Can you work these out from the model? Positions are in its coordinate system, mm. Round coordinates to 2 decimals unless told otherwise and drop trailing zeros. Write each loop counter-clockwise with the first axis right and the second up, starting at its lowest first coordinate (ties: lowest second). Pieces come first, ordered by that corner, then holes.
Q1. If we section it at C-C (z = -19): Please give me the cut outline in (x, y), plus the area to 3 significant figures.
Q2. Please list where these lines run through material, in increasing order: line 1 along Z through (x, y) = (-144, 0) (3 decimals); line 2 along Y through (x, z) = (0, -89).
Q3. If we section it at B-B (z = -63): Please give me the cut outline in (x, y), plus the area to 3 significant figures.
Q4. I'm going to push flat-ended pins straight in: pin 1 Ø1 at (y, z) = (110, -17.5) entering from -X; pin 2 Ø1.5 at (y, z) = (65.5, -40) entering from -X; pin 3 Ø10 at (y, z) = (0, -31.75) entering from -X (3 decimals). Where does each tip first touch, or does it pass through?
from build123d import *

# Parameters (mm, degrees)
BOSS_EXTRUDE2_REACH = 98.52
SKETCH10_R          = 25.4
SKETCH11_R          = 12.7
CUT_EXTRUDE1_DEPTH  = 190.754
CIRPATTERN1_COUNT   = 6


with BuildPart() as part:
    # Sketch1 → Revolve1 (revolve)
    with BuildSketch(Plane(origin=(0, 0, 0), x_dir=(1, 0, 0), z_dir=(0, 1, 0))):
        with BuildLine():
            Line((-148.59, 0), (-140.97, 0))
            Line((-140.97, 0), (-140.97, 12.391039743))
            ThreePointArc((-140.97, 12.391039743), (-134.615921102, 34.866271953), (-117.434796957, 50.687755913))
            ThreePointArc((-117.434796957, 50.687755913), (-60.367509579, 71.617582047), (0, 78.72368491))
            Line((0, 78.72368491), (0, 85.07368491))
            ThreePointArc((0, 85.07368491), (-61.842045719, 77.794008454), (-120.303258046, 56.352950612))
            ThreePointArc((-120.303258046, 56.352950612), (-131.462846302, 48.602983737), (-140.081763243, 38.1))
            Line((-140.081763243, 38.1), (-149.225, 38.1))
            Line((-149.225, 38.1), (-149.225, 25.4))
            Line((-149.225, 25.4), (-152.4, 25.4))
            Line((-152.4, 25.4), (-156.21, 13.674025723))
            Line((-156.21, 13.674025723), (-156.21, 9.503030405))
            Line((-156.21, 9.503030405), (-152.4, 12.7))
            Line((-152.4, 12.7), (-148.59, 12.7))
            Line((-148.59, 12.7), (-148.59, 0))
        make_face()
    revolve(axis=Axis((0, 0, -78.72368491), (0, 0, -1)))

    # Sketch10 → Boss-Extrude2 (add, up to next)
    with BuildSketch(Plane.XY.offset(-96.52), mode=Mode.PRIVATE) as boss_extrude2_sk1:
        Circle(SKETCH10_R)
    boss_extrude2_tool1 = extrude(boss_extrude2_sk1.sketch, amount=BOSS_EXTRUDE2_REACH, mode=Mode.PRIVATE) - part.part
    add(boss_extrude2_tool1.solids().sort_by_distance((0, 0, -96.52))[0])

    # Sketch11 → Cut-Extrude1 (cut)
    with BuildSketch(Plane.XY):
        Circle(SKETCH11_R)
    extrude(amount=-CUT_EXTRUDE1_DEPTH, mode=Mode.SUBTRACT)

    # Sketch15 → 1/4 (0.25) Diameter Hole1 (revolve, cut)
    with BuildSketch(Plane(origin=(149.225, 0, -31.75), x_dir=(0, 0, -1), z_dir=(0, 1, 0))):
        Polygon((0, 0), (0, 8.257732465), (3.175, 6.35), (3.175, 0), align=None)
    f_1_4_0_25_diameter_hole1 = revolve(axis=Axis((155.575, 0, -31.75), (-1, 0, 0)), mode=Mode.SUBTRACT)

    # CirPattern1: 1/4 (0.25) Diameter Hole1 ×6 about axis
    cirpattern1_axis = Axis((0, 0, 5.473137056), (0, 0, -1))
    for i in range(1, CIRPATTERN1_COUNT):
        add(f_1_4_0_25_diameter_hole1.rotate(cirpattern1_axis, i * 360 / CIRPATTERN1_COUNT), mode=Mode.SUBTRACT)


solid = part.part
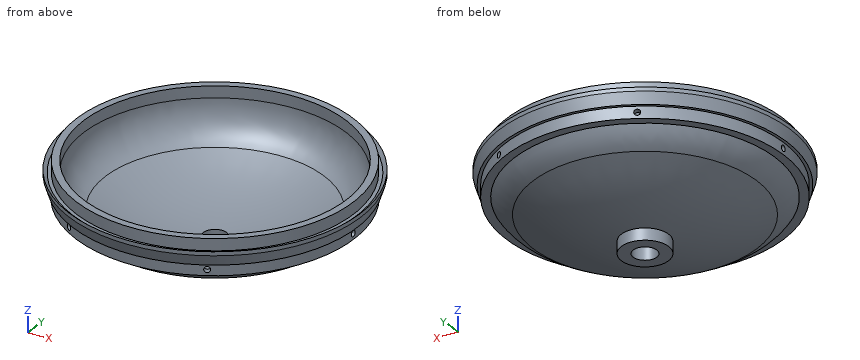
A:
1. outline: circle Ø308.96 at (0, 0); hole circle Ø280.92 at (0, 0)
1. area: 13,000 mm2
2. line 1: z = -38.1 to -34.925, -28.575 to 0
2. line 2: y = -25.4 to -12.7, 12.7 to 25.4
3. outline: circle Ø212.32 at (0, 0); hole circle Ø178.08 at (0, 0)
3. area: 10,500 mm2
4. pin 1: stops at x = -109.71
4. pin 2: stops at x = -123.13
4. pin 3: stops at x = -149.225
